CAD build for the part. Positions are in the model's coordinates, mm. A direction names the side the tool comes from. Round coordinates to 2 decimals unless told otherwise and drop trailing zeros. Loops run counter-clockwise (first coordinate to the right, second up) from the corner with the lowest first, then second, coordinate; pieces in that order, holes last.
Autodesk Inventor part; units mm, degrees
ref_plane "YZ Plane" through (0, 0, 0) normal (1, 0, 0) x (0, 1, 0)
ref_plane "XZ Plane" through (0, 0, 0) normal (0, 1, 0) x (-1, 0, 0)
ref_plane "XY Plane" through (0, 0, 0) normal (0, 0, 1) x (1, 0, 0)
sketch "Szkic1" plane through (0, 0, 0) normal (0, 1, 0) x (-1, 0, 0)
  circle A0 centre (0, 0) radius 12.5
  dimension "d0" = 25
extrude "Wyciągnięcie proste1" add sketch "Szkic1" along normal blind 40
fillet "Zaokrąglenie1" radius 4 1 edges at (12.5, 0, 0)
sketch "Szkic2" plane through (0, 40, 0) normal (0, 1, 0) x (1, 0, 0)
  circle A0 centre (0, 0) radius 12.5
  circle A1 centre (0, 0) radius 8
  dimension "d4" = 16
extrude "Wyciągnięcie proste2" cut sketch "Szkic2" against normal blind 20 contours A1
sketch "Szkic3" plane through (0, 20, 0) normal (0, 1, 0) x (1, 0, 0)
  circle A0 centre (0, 0) radius 8
  circle A1 centre (0, 0) radius 4.5
  dimension "d7" = 9
extrude "Wyciągnięcie proste3" cut sketch "Szkic3" against normal blind 6 contours A1
chamfer "Faza1" distance 0.5 angle 45 1 edges at (-4.5, 20, 0)
properties part number "koncowka do laski - walec zaokraglony"
Item 1: Wall check: L1, parallel to Z at x = 0, y = 18; L2, parallel to Y at x = 5.5, z = -5.5; L3, parallel to X at y = 17, z = -3.25. Give the ranges that are in metal, low to high.
Verdict:
L1: z = -12.5 to -4.5, 4.5 to 12.5
L2: y = 0 to 20
L3: x = -12.07 to -3.11, 3.11 to 12.07
Item 2: Cut at D-D (y = 5). List the corners of the cut face in (x, z), plus the area to 3 significant figures.
Verdict:
outline: circle Ø25 at (0, 0)
area: 491 mm2
Item 3: Flat gauge pins, fed straight in: P1, Ø2, axis at y = 35, z = -6, coming from the +X side; P2, Ø8, axis at x = 9.5, z = -4, coming from the -Y side; P3, Ø4, axis at x = -6.5, y = 24, coming from the -Z side; P4, Ø5.5, axis at x = 0, z = 0, coming from the +Y side. Where does each tip first touch, or does it go through?
Verdict:
P1: stops at x = 11.46
P2: stops at y = 0
P3: stops at z = -11.66
P4: stops at y = 14
Item 4: Cut at B-B (y = 35.5). List the corners of the cut face in (x, z).
Verdict:
outline: circle Ø25 at (0, 0); hole circle Ø16 at (0, 0)
Item 5: Mould opens along X. For faces 1 (the flat face through (0.2, 40, -8.2)), 2 (the cylindrical face through (-1.73, 30.14, 7.81)), 3 (the cylindrical face through (-11.923, 21.748, -3.755)) say: released by +X, released by -X, zero draft, split by the parting line, or undercut.
Verdict:
face 1: zero draft
face 2: undercut
face 3: split by the parting line
Item 6: Cut at C-C (x = 0). List the corners of the cut face in (y, z), plus the area to 3 significant figures.
Verdict:
outline: (0, -8.5) arc R4 ccw to (4, -12.5) - (40, -12.5) - (40, -8) - (20, -8) - (20, -5) - (19.5, -4.5) - (14, -4.5) - (14, 4.5) - (19.5, 4.5) - (20, 5) - (20, 8) - (40, 8) - (40, 12.5) - (4, 12.5) arc R4 ccw to (0, 8.5) - close
area: 619 mm2
Item 7: Cut at A-A (z = 0). List the corners of the cut face in (x, y), plus the area to 3 significant figures.
Verdict:
outline: (-12.5, 4) arc R4 ccw to (-8.5, 0) - (8.5, 0) arc R4 ccw to (12.5, 4) - (12.5, 40) - (8, 40) - (8, 20) - (5, 20) - (4.5, 19.5) - (4.5, 14) - (-4.5, 14) - (-4.5, 19.5) - (-5, 20) - (-8, 20) - (-8, 40) - (-12.5, 40) - close
area: 619 mm2
Item 8: 3-axis set-ups, long thin cutter, end or side, ignore diameter. For faces 4 (the flat face through (0, 0, 0)), 5 (the cylindrical face through (-0.59, 16.79, -4.46)): which of +Z, -Z, +X, -X, +Y, -Y reach the whole face in a straight line?
Verdict:
face 4: +Z, -Z, +X, -X, -Y
face 5: +Y
